```python
from build123d import *

# Parameters (mm, degrees)
F0_W     = 127
F0_H     = 76.2
F1_DEPTH = 63.5
F2_W     = 76.2
F2_H     = 25.4
F3_DEPTH = 75.184
F4_W     = 111.76
F4_H     = 48.26
F5_DEPTH = 86.868
F6_R     = 6.35
F7_DEPTH = 142.748


with BuildPart() as f1:
    # F0 (on Front) → F1 (new body)
    with BuildSketch(Plane.XZ):
        Rectangle(F0_W, F0_H)
    extrude(amount=F1_DEPTH)

    # F2 (on face) → F3 (cut)
    with BuildSketch(Plane.XZ.offset(63.5)):
        with Locations((0, 25.4)):
            Rectangle(F2_W, F2_H)
    extrude(amount=-F3_DEPTH, mode=Mode.SUBTRACT)

    # F4 (on face) → F5 (cut)
    with BuildSketch(Plane.XY.offset(38.1)):
        with Locations((0, -31.75)):
            Rectangle(F4_W, F4_H)
    extrude(amount=-F5_DEPTH, mode=Mode.SUBTRACT)

    # F6 (on face) → F7 (cut)
    with BuildSketch(Plane.YZ.offset(63.5)):
        with Locations((-33.02, -17.78)):
            Circle(F6_R)
    extrude(amount=-F7_DEPTH, mode=Mode.SUBTRACT)


solid = f1.part
```
Here's how the part is built. I have some questions about the finished solid (model axes, mm). A direction names the side the tool comes from. Coordinates: 2 decimals unless noted, no trailing zeros. Order: outer loops, then holes, each group sorted by start corner. A loop starts at its lowest first (then second) coordinate and runs counter-clockwise, first axis right, second up. Notation, with made-up numbers: M -23,2 L 17,2 A19 ccw 17,25 Z; hole C -35.75,83.25 d10. An arc over 180 degrees is marked long. Answer as a JSON object with one key per item and string values. Group by question number.
(1) If we mould it in two halves opening along Z, with no side actions, what happens to faces 4 (the face through (59.74, -38.06, -21.64)), 5 (the face through (-1, 0, -8)), 6 (the face through (0, -6, -38.1))? For each: released by +Z, released by -Z, zero draft, split by the parting line, or undercut.
(2) Suppose I cut it at B-B, the plane x = 40. Please give me the cut outline in (y, z).
(3) For pin 1 (4 mm diameter, centred on x = -11, y = -2.5, fed in from +Z), with a flat end and sliding along its axis, tell me the tip position at first contact or that it passes through.
(4) Suppose I cut it at C-C, the plane y = -50. Please give me the cut outline in (x, z).
(5) I need wall thicknesses on probe 1 along X at (y, z) = (-54.5, -14); probe 2 along Y at (x, z) = (45, -2.5); probe 3 along Z at (x, y) = (-58.5, -33.02). Which ranges of each line are inside material? Lowest first, please.
(6) Suppose I cut it at D-D, the plane z = 11. Please give me the cut outline in (x, y).
(7) Which directions (+Z, -Z, +X, -X, +Y, -Y) give clear straight access to the entire face, cutting with the end or side of a thin tool? Please do faces 1 (the face through (38.1, -60, 25)), 2 (the face through (-59.64, -38.06, -21.64)), 3 (the face through (-1, -7.62, -8)).
(8) Suppose I cut it at A-A, the plane z = 27.5. Please give me the cut outline in (x, y), then the cut area to 3 significant figures.
Values found:
{
 "1": {"face 4": "undercut", "face 5": "zero draft", "face 6": "released by -Z"},
 "2": {"outline": "M -63.5,-38.1 L -55.88,-38.1 L -55.88,38.1 L -63.5,38.1 Z; M -7.62,-38.1 L 0,-38.1 L 0,38.1 L -7.62,38.1 Z"},
 "3": {"pin 1": "stops at z = 12.7"},
 "4": {"outline": "M -63.5,-38.1 L -55.88,-38.1 L -55.88,38.1 L -63.5,38.1 Z; M 55.88,-38.1 L 63.5,-38.1 L 63.5,38.1 L 55.88,38.1 Z"},
 "5": {"probe 1": "x = -63.5 to -55.88, 55.88 to 63.5", "probe 2": "y = -63.5 to -55.88, -7.62 to 0", "probe 3": "z = -38.1 to -24.13, -11.43 to 38.1"},
 "6": {"outline": "M -63.5,-63.5 L 63.5,-63.5 L 63.5,0 L -63.5,0 Z; hole M -55.88,-55.88 L 55.88,-55.88 L 55.88,-7.62 L -55.88,-7.62 Z"},
 "7": {"face 1": "+Z, +Y, -Y", "face 2": "+X, -X", "face 3": "+Z, -Z"},
 "8": {"outline": "M -63.5,-63.5 L -38.1,-63.5 L -38.1,-55.88 L -55.88,-55.88 L -55.88,-7.62 L -38.1,-7.62 L -38.1,0 L -63.5,0 Z; M 38.1,-63.5 L 63.5,-63.5 L 63.5,0 L 38.1,0 L 38.1,-7.62 L 55.88,-7.62 L 55.88,-55.88 L 38.1,-55.88 Z", "area": "1,510 mm^2"}
}
